Work out the finished part from the listing and answer in its coordinate system (mm). Face numbers are marked on the shaded views. A direction names the side the tool comes from. Round coordinates to 2 decimals unless told otherwise and drop trailing zeros. Write each loop counter-clockwise with the first axis right and the second up, starting at its lowest first coordinate (ties: lowest second). Pieces come first, ordered by that corner, then holes.
1. Determine the mould class of the marked faces 1, 2 and 3 for opening direction X: pulls with the +X half, pulls with the -X half, needs draft (parallel to the pull), parting line crosses it, or undercut.
2. Flat-ended cylindrical pins translate along their axes: pin 1 Ø10 at (x, z) = (-34, 15) entering from +Y; pin 2 Ø7.5 at (x, z) = (12.5, 8) entering from -Y. Find the tip coordinate at first contact, or state that the pin passes through.
3. Find section A-A (x = 0). Write down the section's boundary in (y, z), and give its area (3 significant figures).
4. Find section C-C (z = 20.5). Write down the section's boundary in (x, y), and give its area (3 significant figures).
5. A tool of negligible diameter and unlimited length cuts with its end or side. For the marked faces 4 and 5, from which of +Z, -Z, +X, -X, +Y, -Y can it reach the whole face along a straight path? Write none if from no direction.
6. Straight lines are drawn through the part: probe 1 along Y at (x, z) = (0, 20); probe 2 along X at (y, z) = (-26, 16); probe 3 along X at (y, z) = (80, 17.75). For each, find the intervals that lie inside material, in ascending order.
7. Find section B-B (y = 35.5). Write down the section's boundary in (x, z).
8. Find section D-D (y = 113). Write down the section's boundary in (x, z), and give its area (3 significant figures).
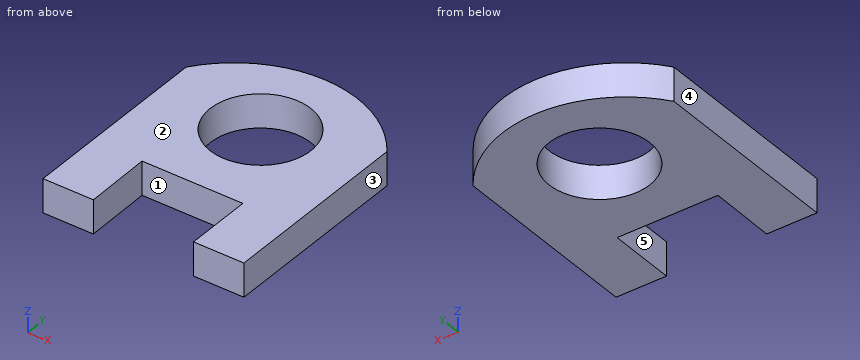
```python
from build123d import *

# Parameters (mm, degrees)
F1_DEPTH = 25.4
F3_D     = 76.2


with BuildPart() as f1:
    # F0 (on Top) → F1 (new body)
    with BuildSketch(Plane.XY):
        with BuildLine():
            Line((-37.8053453803, -50.8), (-38.3331997294, 0))
            Line((-38.3331997294, 0), (37.8668002706, 0))
            Line((37.8668002706, 0), (37.8668002706, -50.8))
            Line((37.8668002706, -50.8), (75.9668002706, -50.8))
            Line((75.9668002706, -50.8), (75.9668002706, 0))
            Line((75.9668002706, 0), (75.9668002706, 96.52))
            ThreePointArc((75.9668002706, 96.52), (0.0307274451, 135.6912791975), (-75.9053453803, 96.52))
            Line((-75.9053453803, 96.52), (-75.9053453803, 0))
            Line((-75.9053453803, 0), (-75.9053453803, -50.8))
            Line((-75.9053453803, -50.8), (-37.8053453803, -50.8))
        make_face()
    extrude(amount=F1_DEPTH)

    # F3 (through all)
    with Locations(Plane(origin=(0, 0, 0), x_dir=(1, 0, 0), z_dir=(0, 0, -1))):
        with Locations((0, -69.78520751)):
            Hole(F3_D / 2)


solid = f1.part
```
Worked answers:
1. face 1: undercut
1. face 2: needs draft
1. face 3: pulls with the +X half
2. pin 1: stops at y = 131.05
2. pin 2: stops at y = 0
3. outline: (0, 0) - (31.69, 0) - (31.69, 25.4) - (0, 25.4) - close; (107.89, 0) - (135.69, 0) - (135.69, 25.4) - (107.89, 25.4) - close
3. area: 1,510 mm2
4. outline: (-75.91, -50.8) - (-37.81, -50.8) - (-38.33, 0) - (37.87, 0) - (37.87, -50.8) - (75.97, -50.8) - (75.97, 96.52) arc R93.19 ccw to (-75.91, 96.52) - close; hole circle Ø76.2 at (0, 69.79)
4. area: 18,100 mm2
5. face 4: +Z, -Z, -X, +Y, -Y
5. face 5: +Z, -Z, -Y
6. probe 1: y = 0 to 31.69, 107.89 to 135.69
6. probe 2: x = -75.91 to -38.06, 37.87 to 75.97
6. probe 3: x = -75.91 to -36.71, 36.71 to 75.97
7. outline: (-75.91, 0) - (-16.62, 0) - (-16.62, 25.4) - (-75.91, 25.4) - close; (16.62, 0) - (75.97, 0) - (75.97, 25.4) - (16.62, 25.4) - close
8. outline: (-60.91, 0) - (60.98, 0) - (60.98, 25.4) - (-60.91, 25.4) - close
8. area: 3,100 mm2
